```python
from build123d import *

# Parameters (mm, degrees)
PARED_DEPTH             = 23
CONECTORES_REACH        = 154.052
CROQUIS2_W              = 16
CROQUIS2_H              = 13
CROQUIS2_W_2            = 10
CROQUIS2_H_2            = 4
CROQUIS2_H_3            = 7
BASE_START              = -1.12
BASE_FRENTE_DEPTH       = 1.12
LUCES_REACH             = 153.399
CROQUIS3_R              = 1.5
CROQUIS3_R_2            = 2.5
SALIENTE_EXTRUIR1_START = 12
CROQUIS3_3_R            = 2.3
CROQUIS3_3_R_2          = 1.5
SALIENTE_EXTRUIR1_DEPTH = 12
SALIENTE_EXTRUIR2_START = 9
CROQUIS3_4_R            = 3.3
CROQUIS3_4_R_2          = 2.5
SALIENTE_EXTRUIR2_DEPTH = 9
SALIENTE_EXTRUIR3_START = 6
CROQUIS3_5_R            = 2.3
CROQUIS3_5_R_2          = 1.5
SALIENTE_EXTRUIR3_DEPTH = 6
SALIENTE_EXTRUIR4_DEPTH = 12
CROQUIS5_W              = 2
CROQUIS5_H              = 0.8
SALIENTE_EXTRUIR5_DEPTH = 0.4
CHAFL_N1_SIZE           = 0.4
CHAFL_N1_SIZE_2         = 0.857802768


with BuildPart() as part:
    # Croquis1 → pared (new body)
    with BuildSketch(Plane.XY):
        with BuildLine():
            Line((3, 61.1), (132, 61.1))
            ThreePointArc((132, 61.1), (135.252691193, 59.752691193), (136.6, 56.5))
            Line((136.6, 56.5), (136.6, 3))
            ThreePointArc((136.6, 3), (135.252691193, -0.252691193), (132, -1.6))
            Line((132, -1.6), (3, -1.6))
            ThreePointArc((3, -1.6), (-0.252691193, -0.252691193), (-1.6, 3))
            Line((-1.6, 3), (-1.6, 56.5))
            ThreePointArc((-1.6, 56.5), (-0.252691193, 59.752691193), (3, 61.1))
        make_face()
        with BuildLine():
            Line((3, 0), (132, 0))
            ThreePointArc((132, 0), (134.121320344, 0.878679656), (135, 3))
            Line((135, 3), (135, 56.5))
            ThreePointArc((135, 56.5), (134.121320344, 58.621320344), (132, 59.5))
            Line((132, 59.5), (3, 59.5))
            ThreePointArc((3, 59.5), (0.878679656, 58.621320344), (0, 56.5))
            Line((0, 56.5), (0, 3))
            ThreePointArc((0, 3), (0.878679656, 0.878679656), (3, 0))
        make_face(mode=Mode.SUBTRACT)
    extrude(amount=PARED_DEPTH)

    # Croquis2 → conectores (cut, up to next)
    with BuildSketch(Plane.XZ.offset(1.6), mode=Mode.PRIVATE) as conectores_sk1:
        with Locations((110, 6.5)):
            Rectangle(CROQUIS2_W, CROQUIS2_H)
    conectores_tool1 = extrude(conectores_sk1.sketch, amount=-CONECTORES_REACH, mode=Mode.PRIVATE) & part.part
    # Croquis2 → conectores (cut, up to next)
    with BuildSketch(Plane.XZ.offset(1.6), mode=Mode.PRIVATE) as conectores_sk2:
        with Locations((93, 12.5)):
            Rectangle(CROQUIS2_W_2, CROQUIS2_H_2)
    conectores_tool2 = extrude(conectores_sk2.sketch, amount=-CONECTORES_REACH, mode=Mode.PRIVATE) & part.part
    # Croquis2 → conectores (cut, up to next)
    with BuildSketch(Plane.XZ.offset(1.6), mode=Mode.PRIVATE) as conectores_sk3:
        with Locations((30.5, 3.5)):
            Rectangle(CROQUIS2_W_2, CROQUIS2_H_3)
    conectores_tool3 = extrude(conectores_sk3.sketch, amount=-CONECTORES_REACH, mode=Mode.PRIVATE) & part.part
    add(conectores_tool1.solids().sort_by_distance((110, -1.6, 6.5))[0], mode=Mode.SUBTRACT)
    add(conectores_tool2.solids().sort_by_distance((93, -1.6, 12.5))[0], mode=Mode.SUBTRACT)
    add(conectores_tool3.solids().sort_by_distance((30.5, -1.6, 3.5))[0], mode=Mode.SUBTRACT)

    # Croquis1<2> → base frente (add)
    with BuildSketch(Plane.XY.offset(BASE_START)):
        with BuildLine():
            Line((3, 61.1), (132, 61.1))
            ThreePointArc((132, 61.1), (135.252691193, 59.752691193), (136.6, 56.5))
            Line((136.6, 56.5), (136.6, 3))
            ThreePointArc((136.6, 3), (135.252691193, -0.252691193), (132, -1.6))
            Line((132, -1.6), (3, -1.6))
            ThreePointArc((3, -1.6), (-0.252691193, -0.252691193), (-1.6, 3))
            Line((-1.6, 3), (-1.6, 56.5))
            ThreePointArc((-1.6, 56.5), (-0.252691193, 59.752691193), (3, 61.1))
        make_face()
    extrude(amount=BASE_FRENTE_DEPTH)

    # Croquis3 → luces (cut, up to next)
    with BuildSketch(Plane.XY, mode=Mode.PRIVATE) as luces_sk1:
        with Locations((130.5, 48)):
            Circle(CROQUIS3_R)
    luces_tool1 = extrude(luces_sk1.sketch, amount=-LUCES_REACH, mode=Mode.PRIVATE) & part.part
    # Croquis3 → luces (cut, up to next)
    with BuildSketch(Plane.XY, mode=Mode.PRIVATE) as luces_sk2:
        with Locations((130.5, 41.5)):
            Circle(CROQUIS3_R)
    luces_tool2 = extrude(luces_sk2.sketch, amount=-LUCES_REACH, mode=Mode.PRIVATE) & part.part
    # Croquis3 → luces (cut, up to next)
    with BuildSketch(Plane.XY, mode=Mode.PRIVATE) as luces_sk3:
        with Locations((130.5, 35)):
            Circle(CROQUIS3_R)
    luces_tool3 = extrude(luces_sk3.sketch, amount=-LUCES_REACH, mode=Mode.PRIVATE) & part.part
    # Croquis3 → luces (cut, up to next)
    with BuildSketch(Plane.XY, mode=Mode.PRIVATE) as luces_sk4:
        with Locations((130.5, 28.5)):
            Circle(CROQUIS3_R)
    luces_tool4 = extrude(luces_sk4.sketch, amount=-LUCES_REACH, mode=Mode.PRIVATE) & part.part
    # Croquis3 → luces (cut, up to next)
    with BuildSketch(Plane.XY, mode=Mode.PRIVATE) as luces_sk5:
        with Locations((130.5, 17.5)):
            Circle(CROQUIS3_R)
    luces_tool5 = extrude(luces_sk5.sketch, amount=-LUCES_REACH, mode=Mode.PRIVATE) & part.part
    # Croquis3 → luces (cut, up to next)
    with BuildSketch(Plane.XY, mode=Mode.PRIVATE) as luces_sk6:
        with Locations((130.5, 11.5)):
            Circle(CROQUIS3_R_2)
    luces_tool6 = extrude(luces_sk6.sketch, amount=-LUCES_REACH, mode=Mode.PRIVATE) & part.part
    # Croquis3 → luces (cut, up to next)
    with BuildSketch(Plane.XY, mode=Mode.PRIVATE) as luces_sk7:
        with Locations((3.5, 15)):
            Circle(CROQUIS3_R)
    luces_tool7 = extrude(luces_sk7.sketch, amount=-LUCES_REACH, mode=Mode.PRIVATE) & part.part
    add(luces_tool1.solids().sort_by_distance((130.5, 48, 0))[0], mode=Mode.SUBTRACT)
    add(luces_tool2.solids().sort_by_distance((130.5, 41.5, 0))[0], mode=Mode.SUBTRACT)
    add(luces_tool3.solids().sort_by_distance((130.5, 35, 0))[0], mode=Mode.SUBTRACT)
    add(luces_tool4.solids().sort_by_distance((130.5, 28.5, 0))[0], mode=Mode.SUBTRACT)
    add(luces_tool5.solids().sort_by_distance((130.5, 17.5, 0))[0], mode=Mode.SUBTRACT)
    add(luces_tool6.solids().sort_by_distance((130.5, 11.5, 0))[0], mode=Mode.SUBTRACT)
    add(luces_tool7.solids().sort_by_distance((3.5, 15, 0))[0], mode=Mode.SUBTRACT)

    # Croquis3<3> → Saliente-Extruir1 (add)
    # profile 1 of 5: a face of its own
    with BuildSketch(Plane.XY.offset(SALIENTE_EXTRUIR1_START)):
        with Locations((130.5, 17.5)):
            Circle(CROQUIS3_3_R)
        with Locations((130.5, 17.5)):
            Circle(CROQUIS3_3_R_2, mode=Mode.SUBTRACT)
    # profile 2 of 5: a face of its own
    with BuildSketch(Plane.XY.offset(SALIENTE_EXTRUIR1_START)):
        with Locations((130.5, 28.5)):
            Circle(CROQUIS3_3_R)
        with Locations((130.5, 28.5)):
            Circle(CROQUIS3_3_R_2, mode=Mode.SUBTRACT)
    # profile 3 of 5: a face of its own
    with BuildSketch(Plane.XY.offset(SALIENTE_EXTRUIR1_START)):
        with Locations((130.5, 35)):
            Circle(CROQUIS3_3_R)
        with Locations((130.5, 35)):
            Circle(CROQUIS3_3_R_2, mode=Mode.SUBTRACT)
    # profile 4 of 5: a face of its own
    with BuildSketch(Plane.XY.offset(SALIENTE_EXTRUIR1_START)):
        with Locations((130.5, 41.5)):
            Circle(CROQUIS3_3_R)
        with Locations((130.5, 41.5)):
            Circle(CROQUIS3_3_R_2, mode=Mode.SUBTRACT)
    # profile 5 of 5: a face of its own
    with BuildSketch(Plane.XY.offset(SALIENTE_EXTRUIR1_START)):
        with Locations((130.5, 48)):
            Circle(CROQUIS3_3_R)
        with Locations((130.5, 48)):
            Circle(CROQUIS3_3_R_2, mode=Mode.SUBTRACT)
    extrude(amount=-SALIENTE_EXTRUIR1_DEPTH)

    # Croquis3<4> → Saliente-Extruir2 (add)
    with BuildSketch(Plane.XY.offset(SALIENTE_EXTRUIR2_START)):
        with Locations((130.5, 11.5)):
            Circle(CROQUIS3_4_R)
        with Locations((130.5, 11.5)):
            Circle(CROQUIS3_4_R_2, mode=Mode.SUBTRACT)
    extrude(amount=-SALIENTE_EXTRUIR2_DEPTH)

    # Croquis3<5> → Saliente-Extruir3 (add)
    with BuildSketch(Plane.XY.offset(SALIENTE_EXTRUIR3_START)):
        with Locations((3.5, 15)):
            Circle(CROQUIS3_5_R)
        with Locations((3.5, 15)):
            Circle(CROQUIS3_5_R_2, mode=Mode.SUBTRACT)
    extrude(amount=-SALIENTE_EXTRUIR3_DEPTH)

    # Croquis4 → Saliente-Extruir4 (add)
    with BuildSketch(Plane.XY):
        Polygon((36.5, 0), (36.5, 0.6), (35.5, 0.6), (35.5, 1.4), (37.1, 1.4), (38, 0), align=None)
        Polygon((24.5, 0), (23, 0), (23.9, 1.4), (25.5, 1.4), (25.5, 0.6), (24.5, 0.6), align=None)
    extrude(amount=SALIENTE_EXTRUIR4_DEPTH)

    # Croquis5 → Saliente-Extruir5 (add)
    with BuildSketch(Plane(origin=(0, 0, 0), x_dir=(1, 0, 0), z_dir=(0, 1, 0))):
        with Locations((30.5, -12.4)):
            Rectangle(CROQUIS5_W, CROQUIS5_H)
    extrude(amount=SALIENTE_EXTRUIR5_DEPTH)

    # Chaflán1
    # the kernel refuses this chamfer: 0.857802768, 0.4 mm, written as the material it takes off along each edge
    with BuildSketch(Plane(origin=(27.277454068, 0.4, 12.8), x_dir=(0, -0.9971975577536771, 0.07481330637060238), z_dir=(1, 0, 0))) as chafl_n1_piece_1_section:
        Polygon((CHAFL_N1_SIZE * 0.997197557754, CHAFL_N1_SIZE * 0.0748133063706), (-CHAFL_N1_SIZE_2 * 0.0748133063884, CHAFL_N1_SIZE_2 * 0.997197557991), (0, 0), align=None)
    chafl_n1_piece_1 = extrude(amount=6.445091863, mode=Mode.PRIVATE)
    chafl_n1_piece_1 = split(chafl_n1_piece_1, bisect_by=Plane(origin=(30.5, 0, 12.509130299), z_dir=(0, 1, 0)), keep=Keep.TOP, mode=Mode.PRIVATE)
    add(chafl_n1_piece_1, mode=Mode.SUBTRACT)


solid = part.part
```
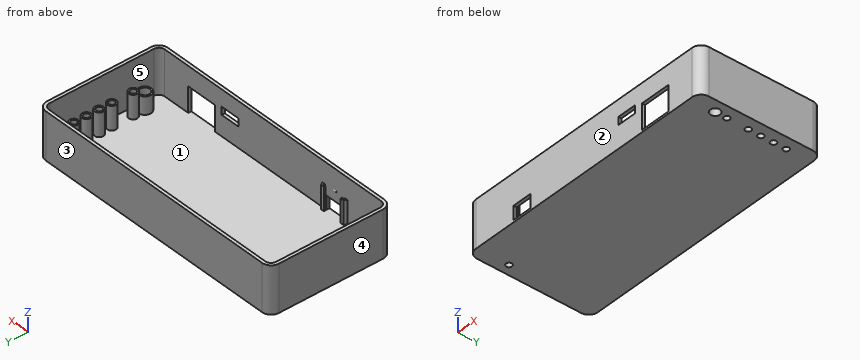
Geometry check sheet. Reference: the model listing, model coordinates, mm. Face numbers are marked on the shaded views. A direction names the side the tool comes from. Round coordinates to 2 decimals unless told otherwise and drop trailing zeros. Loops run counter-clockwise (first coordinate to the right, second up) from the corner with the lowest first, then second, coordinate; pieces in that order, holes last. Notation, with made-up numbers: (13, 13) -> (51, 13) arc R27 cw to (51, 29) -> close; hole circle Ø11 at (52, 20.25). An arc over 180 degrees is marked (long way). Use a Markdown table: item, result.
(1) Sectioned sample at A-A (z = 21). Enter the section's corners in (x, y), then the cut area to 3 significant figures.
Calculated:
| item | result |
|---|---|
| outline | (-1.6, 3) arc R4.6 ccw to (3, -1.6) -> (132, -1.6) arc R4.6 ccw to (136.6, 3) -> (136.6, 56.5) arc R4.6 ccw to (132, 61.1) -> (3, 61.1) arc R4.6 ccw to (-1.6, 56.5) -> close; hole (0, 3) arc R3 ccw to (3, 0) -> (132, 0) arc R3 ccw to (135, 3) -> (135, 56.5) arc R3 ccw to (132, 59.5) -> (3, 59.5) arc R3 ccw to (0, 56.5) -> close |
| area | 622 mm² |
(2) Sectioned sample at B-B (x = 105.5). Enter the section's corners in (y, z).
Calculated:
| item | result |
|---|---|
| outline | (-1.6, -1.12) -> (61.1, -1.12) -> (61.1, 23) -> (59.5, 23) -> (59.5, 0) -> (-1.6, 0) -> close; (-1.6, 13) -> (0, 13) -> (0, 23) -> (-1.6, 23) -> close |
(3) Go/stop test with flat-tipped pins: P1, Ø1.3, axis at y = -1, z = 12, coming from the +X side; P2, Ø0.8, axis at y = -0.5, z = 6.5, coming from the -X side; P3, Ø8, axis at x = 66, y = 33, coming from the +Z side; P4, Ø10, axis at x = 106.5, z = 11, coming from the -Y side. Record where each tip stops, or that it passes through.
Calculated:
| item | result |
|---|---|
| P1 | x = 135.15 |
| P2 | x = -0.4 |
| P3 | z = 0 |
| P4 | y = -1.6 |
(4) Sectioned sample at C-C (y = 35). Enter the section's corners in (x, z).
Calculated:
| item | result |
|---|---|
| outline | (-1.6, -1.12) -> (129, -1.12) -> (129, 12) -> (128.2, 12) -> (128.2, 0) -> (0, 0) -> (0, 23) -> (-1.6, 23) -> close; (132, -1.12) -> (136.6, -1.12) -> (136.6, 23) -> (135, 23) -> (135, 0) -> (132.8, 0) -> (132.8, 12) -> (132, 12) -> close |
(5) Mould release check, pull along Y, two halves, no side actions. Record for the marked faces 1, 2 and 3: released by +Y, released by -Y, zero draft, split by the parting line, or undercut.
Calculated:
| item | result |
|---|---|
| face 1 | undercut |
| face 2 | released by -Y |
| face 3 | released by +Y |
(6) Scan lines: probe 1 along Y at (x, z) = (3.5, 0.5); probe 2 along X at (y, z) = (7, 15); probe 3 along Y at (x, z) = (13, 5.5). Record each from-to range of solid material in increasing order.
Calculated:
| item | result |
|---|---|
| probe 1 | -1.6 to 0, 12.7 to 13.5, 16.5 to 17.3, 59.5 to 61.1 |
| probe 2 | -1.6 to 0, 135 to 136.6 |
| probe 3 | -1.6 to 0, 59.5 to 61.1 |
(7) Set-up check for the marked faces 4 and 5: record each of +Z, -Z, +X, -X, +Y, -Y from which the full face is reachable in a straight line by a thin tool's end or side.
Calculated:
| item | result |
|---|---|
| face 4 | +Z, -Z, -X, +Y, -Y |
| face 5 | +Z |
(8) Sectioned sample at D-D (z = 1.5). Give the number of separate pieces and of enclosed holes in the cut face, then the cut area to 3 significant figures.
Calculated:
| item | result |
|---|---|
| separate pieces | 9 |
| enclosed holes | 7 |
| area | 657 mm² |
